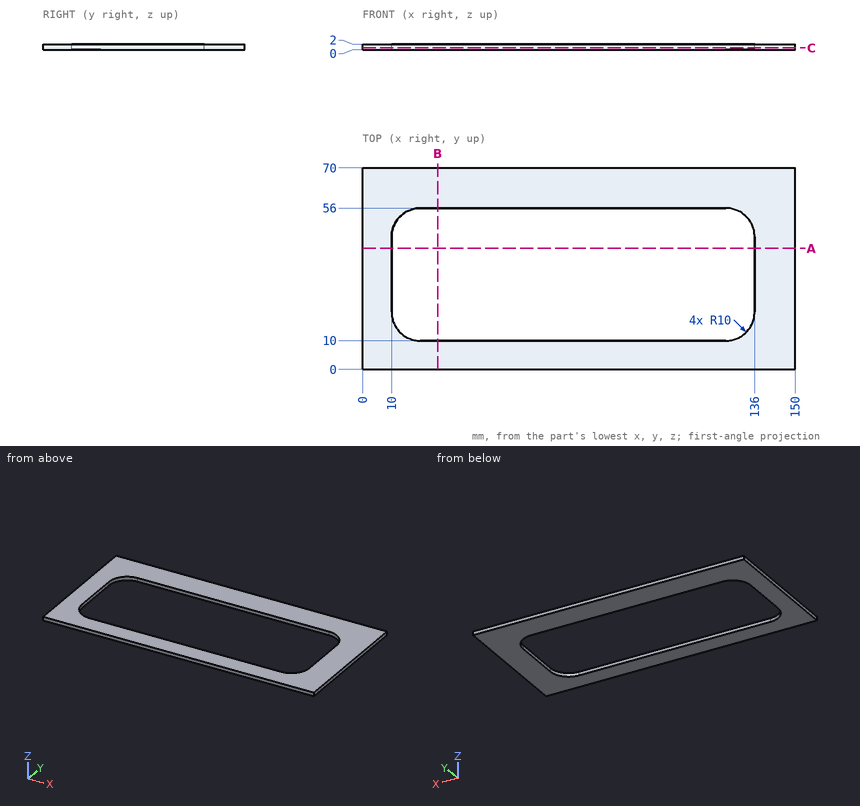
The drawing under review shows one solid part. Ordinate dimensions are in mm from its lowest x, y, z. Give positions to 0.01 mm unless a question says otherwise; leave off trailing zeros. Order: outer loops, then holes, each group sorted by start corner. A loop starts at its lowest first (then second) coordinate and runs counter-clockwise, first axis right, second up. Notation, with made-up numbers: M -18.75,-32.75 L -9.75,-32.75 A26 cw -9.75,-4.75 Z; hole C -24.5,56 d1. An arc over 180 degrees is marked long. One line per question, with ' | ' between items. Start each with the question number.
Q1. For L1, parallel to Y at x = 40.5, z = 0.85; L2, parallel to X at y = 21.5, z = 1.5; L3, parallel to X at y = 11, z = 0.15, list the stretches that pass through material, from the lowest coordinate up. Write a range as [from, to].
Q2. We need section A-A (y = 42). Write out the cut boundary in (x, z).
Q3. For pin 1 Ø12 at (x, y) = (133, 17) entering from +Z, flat-tipped, find the tip position at first contact; note if it passes through.
Q4. We need section C-C (z = 0.65). Write out the cut boundary in (x, y), plus the area to 3 significant figures.
Q5. We need section B-B (x = 26). Write out the cut boundary in (y, z), plus the area to 3 significant figures.
Returned:
1) L1: [0, 10], [56, 70] | L2: [0, 10], [136, 150] | L3: [0, 15.64], [130.36, 150]
2) outline: M 0,0 L 10,0 L 10,2 L 0,2 Z; M 136,0 L 150,0 L 150,2 L 136,2 Z
3) pin 1: z = 2
4) outline: M 0,0 L 150,0 L 150,70 L 0,70 Z; hole M 10,20 A10 ccw 20,10 L 126,10 A10 ccw 136,20 L 136,46 A10 ccw 126,56 L 20,56 A10 ccw 10,46 Z | area: 4,790 mm2
5) outline: M 0,0 L 10,0 L 10,2 L 0,2 Z; M 56,0 L 70,0 L 70,2 L 56,2 Z | area: 48.0 mm2
